The drawing under review shows one solid part. Ordinate dimensions are in mm from its lowest x, y, z. Give positions to 0.01 mm unless a question says otherwise; leave off trailing zeros. Write each loop counter-clockwise with the first axis right and the second up, starting at its lowest first coordinate (ties: lowest second). Pieces come first, ordered by that corner, then holes. Notation, with made-up numbers: (36.25, 52.25) - (77.25, 52.25) arc R23 cw to (77.25, 70.25) - close; hole circle Ø1 at (39.25, 81). An arc over 180 degrees is marked (long way). Write each question's results on one line, items separated by ' | '. Start each with the question number.
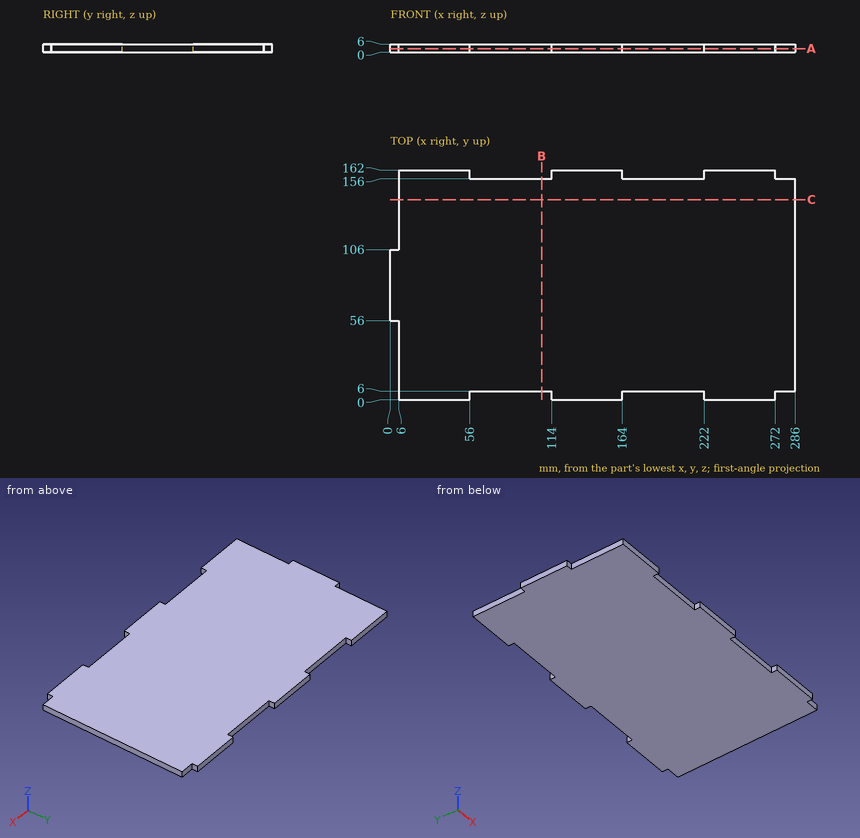
Q1. Insertion check: P1, Ø1.8, axis at y = 4.5, z = 3, coming from the +X side; P2, Ø6, axis at x = 52, y = 128.5, coming from the -Z side; P3, Ø3, axis at x = 185.5, z = 4, coming from the -Y side; P4, Ø1.8, axis at y = 4, z = 3, coming from the -X side. Each pin has a flat end and moves straight along its axis. Give the tip position at first contact, or say it passes through.
Q2. Add section B-B on x = 107. State the section outline as (y, z) points, plus the area to 3 significant figures.
Q3. Add section C-C on y = 141.5. State the section outline as (x, z) points.
Q4. For line 1 along Y through (x, z) = (194, 0.55); line 2 along X through (y, z) = (121, 3.4), list the stretches that pass through material, from the lowest coordinate up. Write a range as [from, to].
Q5. Add section A-A on z = 2.65. State the section outline as (x, y) points.
Result:
1) P1: stops at x = 272 | P2: stops at z = 0 | P3: stops at y = 6 | P4: stops at x = 6
2) outline: (6, 0) - (156, 0) - (156, 6) - (6, 6) - close | area: 900 mm²
3) outline: (6, 0) - (286, 0) - (286, 6) - (6, 6) - close
4) line 1: y = [6, 156] | line 2: x = [6, 286]
5) outline: (0, 56) - (6, 56) - (6, 0) - (56, 0) - (56, 6) - (114, 6) - (114, 0) - (164, 0) - (164, 6) - (222, 6) - (222, 0) - (272, 0) - (272, 6) - (286, 6) - (286, 156) - (272, 156) - (272, 162) - (222, 162) - (222, 156) - (164, 156) - (164, 162) - (114, 162) - (114, 156) - (56, 156) - (56, 162) - (6, 162) - (6, 106) - (0, 106) - close
